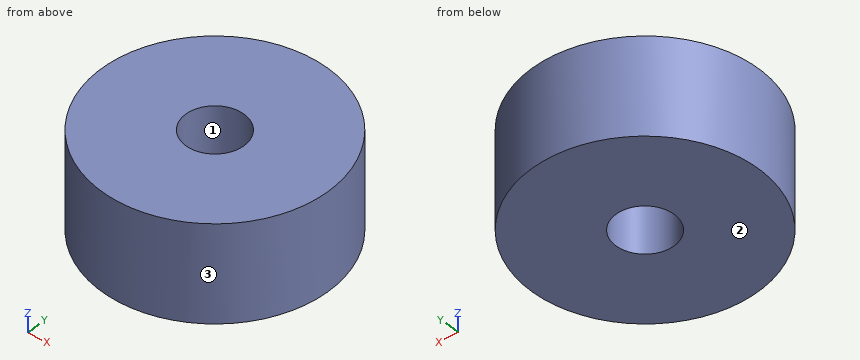
from build123d import *

# Parameters (mm, degrees)
SKETCH1_R           = 350
SKETCH1_R_2         = 90
BOSS_EXTRUDE1_DEPTH = 300
SHELL1_T            = 5


with BuildPart() as part:
    # Sketch1 → Boss-Extrude1 (new body)
    with BuildSketch(Plane.XY):
        Circle(SKETCH1_R)
        Circle(SKETCH1_R_2, mode=Mode.SUBTRACT)
    extrude(amount=BOSS_EXTRUDE1_DEPTH)

    # Shell1 (no face opened: a closed hollow body)
    add(offset(amount=-SHELL1_T, mode=Mode.PRIVATE), mode=Mode.SUBTRACT)


solid = part.part
Input: part model. Units: mm. Frame: model coordinates. Face numbers are marked on the shaded views. Coordinates: 2 decimals unless noted, no trailing zeros. Order: outer loops, then holes, each group sorted by start corner. A loop starts at its lowest first (then second) coordinate and runs counter-clockwise, first axis right, second up. Notation, with made-up numbers: M -9,44.5 L 7,44.5 A10 ccw 7,53.5 Z; hole C 37.5,19 d11. An arc over 180 degrees is marked long. Write item = value, one per line. Start each with the question number.
(1) Section A-A on x = 0. Output: boundary loops of the cut face in (y, z), and give its area (3 significant figures).
(2) Section D-D on y = -273. Output: boundary loops of the cut face in (x, z).
(3) Section C-C on z = 131. Output: boundary loops of the cut face in (x, y).
(4) Line query: line 1 along Y through (x, z) = (0, 76); line 2 along Z through (x, y) = (-246, -211); line 3 along X through (y, z) = (26, 215.5). Output: solid intervals per line, ascending. Write a range as [from, to].
(5) Pull-direction query (X, two-part tool) for the marked faces 1, 2 and 3; classes: released by +X, released by -X, zero draft, split by the parting line, or undercut.
(6) First-contact query: P1, Ø10, axis at x = -50.5, z = 213, coming from the +Y side; P2, Ø10, axis at y = 118.5, z = 60.5, coming from the +X side; P3, Ø5, axis at x = -266, z = 219.5, coming from the -Y side. Flat tips, straight axial feed; report the tip coordinate or a pass-through.
Result set:
q1.outline = M -350,0 L -90,0 L -90,300 L -350,300 Z; M 90,0 L 350,0 L 350,300 L 90,300 Z; hole M -345,5 L -95,5 L -95,295 L -345,295 Z; hole M 95,5 L 345,5 L 345,295 L 95,295 Z
q1.area = 11,000 mm²
q2.outline = M -219.02,0 L 219.02,0 L 219.02,300 L -219.02,300 Z; hole M -210.94,5 L 210.94,5 L 210.94,295 L -210.94,295 Z
q3.outline = C 0,0 d700; C 0,0 d190; hole C 0,0 d690; hole C 0,0 d180
q4.line_1 = [-350, -345], [-95, -90], [90, 95], [345, 350]
q4.line_2 = [0, 5], [295, 300]
q4.line_3 = [-349.03, -344.02], [-91.37, -86.16], [86.16, 91.37], [344.02, 349.03]
q5.face_1 = undercut
q5.face_2 = zero draft
q5.face_3 = split by the parting line
q6.P1 = 347.03
q6.P2 = 331.09
q6.P3 = -230.36
